The listing builds one solid part. Answer for the finished solid, in the listing's coordinates (mm). Face numbers are marked on the shaded views. A direction names the side the tool comes from. Round coordinates to 2 decimals unless told otherwise and drop trailing zeros. Write each loop counter-clockwise with the first axis right and the second up, starting at its lowest first coordinate (ties: lowest second). Pieces come first, ordered by that corner, then holes.
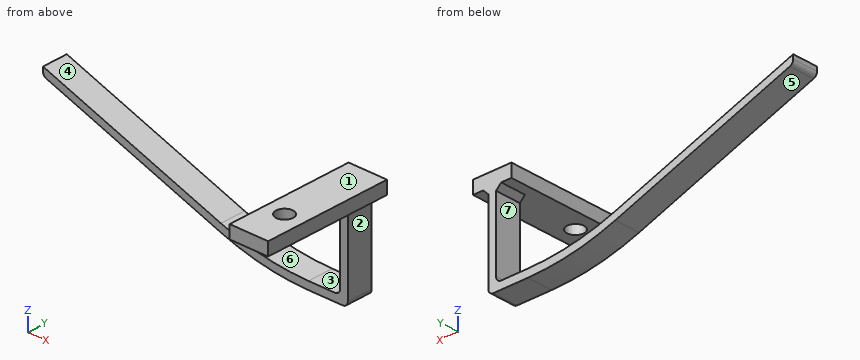
Autodesk Inventor part; units mm, degrees
ref_plane "YZ Plane" through (0, 0, 0) normal (1, 0, 0) x (0, 1, 0)
ref_plane "XZ Plane" through (0, 0, 0) normal (0, 1, 0) x (-1, 0, 0)
ref_plane "XY Plane" through (0, 0, 0) normal (0, 0, 1) x (1, 0, 0)
sketch "Náčrt1" plane through (0, 0, 0) normal (0, 0, 1) x (1, 0, 0)
  line L0 (0, 21) -> (0, -21)
  line L1 (-10.5, 0) -> (10.5, 0)
  line L2 (-7.5, 15) -> (7.5, 15)
  line L3 (7.5, 15) -> (7.5, -15)
  line L4 (7.5, -15) -> (-7.5, -15)
  line L5 (-7.5, -15) -> (-7.5, 15)
  point P0 (0, 0)
  dimension "d0" = 15
  dimension "d1" = 30
extrude "Vysunutí1" add sketch "Náčrt1" along normal blind 5
sketch "Náčrt2" plane through (-7.5, 15, 0) normal (0, 1, 0) x (1, 0, 0)
  line L0 (7.5, 1) -> (7.5, -6)
  line L1 (18, 0) -> (-3, 0)
  line L2 (15, 0) -> (0, 0)
  line L3 (0, 0) -> (0, -5)
  line L4 (15, -5) -> (0, -5)
  line L5 (15, 0) -> (15, -5)
  line L6 (15, 0) -> (0, 0)
  line L7 (0, 0) -> (15, 0)
  line L8 (15, 0) -> (15, -5)
  line L9 (15, -5) -> (0, -5)
  line L10 (0, -5) -> (0, 0)
  point P0 (7.5, 0)
extrude "Vysunutí2" add sketch "Náčrt2" along normal blind 20
sketch "Náčrt3" plane through (0, 0, 5) normal (0, 0, 1) x (1, 0, 0)
  line L0 (-7.5, -15) -> (7.5, -15)
  line L1 (7.5, -15) -> (7.5, 35)
  line L2 (-7.5, 35) -> (7.5, 35)
  line L3 (-7.5, -15) -> (-7.5, 35)
  line L4 (0, 45) -> (0, -25)
  line L5 (-10.5, 0) -> (10.5, 0)
  point P0 (0, 0)
  point P1 (0, 0)
  dimension "d6" = 15
hole "Díra1" at (0, 0, 5) direction (0, 0, -1) diameter 6.6 end through all
sketch "Náčrt4" plane through (-7.5, 35, 0) normal (0, 1, 0) x (1, 0, 0)
  line L0 (15, -5) -> (15, 0)
  line L1 (15, 0) -> (0, 0)
  line L2 (0, 0) -> (0, -5)
  line L3 (0, -5) -> (15, -5)
  line L4 (6, 0) -> (9, 0)
  line L5 (9, 0) -> (9, 35)
  line L6 (9, 35) -> (6, 35)
  line L7 (6, 35) -> (6, 0)
  line L8 (7.5, 43) -> (7.5, -13)
  line L9 (6, 35) -> (-24, 35)
  line L10 (-24, 35) -> (-24, 32)
  line L11 (-24, 32) -> (6, 32)
  line L12 (6, 32) -> (6, 35)
  line L13 (-24, 35) -> (-110, 3.6986)
  line L14 (-24, 32) -> (-110, 0.6986)
  line L15 (-110, 0.6986) -> (-110, 3.6986)
  point P0 (7.5, 0)
  point P1 (6, 32)
  dimension "d14" = 3
  dimension "d15" = 35
  dimension "d16" = 3
  dimension "d17" = 30
  dimension "d19" = 160
  dimension "d20" = 110
extrude "Vysunutí3" add sketch "Náčrt4" against normal blind 10 contours L1 L8 L6 L5 | L1 L7 L6 L8 | L11 L10 L9 L7 | L14 L15 L13 L10
chamfer "Zkosení1" distance 2 distance2 2 2 edges at (-1.5, 30, 0) (1.5, 30, 0) measured on face at (-6.092, 6.7993, 0)
fillet "Zaoblení2" radius 2 1 edges at (-117.5, 30, -3.6986)
fillet "Zaoblení3" radius 2 2 edges at (1.5, 30, -35) (-1.5, 30, -32)
fillet "Zaoblení4" radius 100 2 edges at (-31.5, 30, -32) (-31.5, 30, -35)
properties part number "srovnavac_3D tisk"
1. For a pull along X with two mould halves and no side action, classify the marked faces 1, 2, 3 and 4 as released by +X, released by -X, zero draft, split by the parting line, or undercut.
Geometry says:
face 1: zero draft
face 2: released by +X
face 3: undercut
face 4: undercut
2. Section C-C on y = -10.5 is taken. Determine the outline of the cut face in (x, z).
Geometry says:
outline: (-7.5, 0) - (7.5, 0) - (7.5, 5) - (-7.5, 5) - close
3. Section A-A on y = 0 is taken. Determine the outline of the cut face in (x, z), plus the area to 3 significant figures.
Geometry says:
outline: (-7.5, 0) - (-3.3, 0) - (-3.3, 5) - (-7.5, 5) - close; (3.3, 0) - (7.5, 0) - (7.5, 5) - (3.3, 5) - close
area: 42.0 mm2
4. Section B-B on z = -18.5 is taken. Determine the outline of the cut face in (x, y).
Geometry says:
outline: (-76.83, 25) - (-68.59, 25) - (-68.59, 35) - (-76.83, 35) - close; (-1.5, 25) - (1.5, 25) - (1.5, 35) - (-1.5, 35) - close
5. Section D-D on x = -27 is taken. Determine the outline of the cut face in (y, z).
Geometry says:
outline: (25, -34.13) - (35, -34.13) - (35, -31.13) - (25, -31.13) - close
6. Straight lines are drawn through the part: line 1 along Y through (x, z) = (0, 2.55); line 2 along X through (y, z) = (0, 3); line 3 along X through (y, z) = (-5.5, 3). For each, find the intervals that lie inside material, in ascending order.
Geometry says:
line 1: y = -15 to -3.3, 3.3 to 35
line 2: x = -7.5 to -3.3, 3.3 to 7.5
line 3: x = -7.5 to 7.5
7. Given pin 1 (10 mm diameter, centred on x = -43, y = 24, fed in from -Z); pin 2 (8 mm diameter, centred on y = 22, z = -6, fed in from +X); pin 3 (17.5 mm diameter, centred on x = -28.5, z = -19, fed in from -Y); pin 4 (10 mm diameter, centred on x = -63, y = 27.5, fed in from -Z), each flat-ended and moving along its own axis, determine where each tip first touches the part or whether it passes through.
Geometry says:
pin 1: stops at z = -32.02
pin 2: stops at x = 1.5
pin 3: passes through
pin 4: stops at z = -25.35
8. A tool of negligible diameter and unlimited length cuts with its end or side. For the marked faces 5, 6 and 7, from which of +Z, -Z, +X, -X, +Y, -Y can it reach the whole face along a straight path? Write none if from no direction.
Geometry says:
face 5: -Z, -X, +Y, -Y
face 6: +Z, +Y, -Y
face 7: +Y, -Y
